For this review, take the finished solid that the model builds, in its own axes (mm). Face numbers are marked on the shaded views. A direction names the side the tool comes from. Coordinates: 2 decimals unless noted, no trailing zeros. Loops run counter-clockwise (first coordinate to the right, second up) from the corner with the lowest first, then second, coordinate; pieces in that order, holes last. Notation, with made-up numbers: (81, -34) -> (85, -34) arc R8 cw to (85, -28) -> close; hole circle Ø7 at (-36.5, 36). An arc over 180 degrees is marked (long way). Answer in a Markdown table with one row per item.
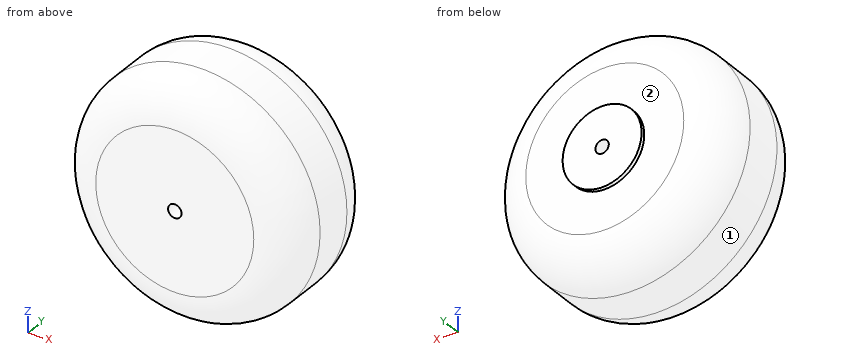
from build123d import *

# Parameters (mm, degrees)
CYLINDER014_R          = 1.7
CYLINDER014_DEPTH      = 31
CYLINDER014_ROLL_ANGLE = 90
CYLINDER012_R          = 30
CYLINDER012_DEPTH      = 30
CYLINDER012_ROLL_ANGLE = 90
CYLINDER013_R          = 10
CYLINDER013_DEPTH      = 31
CYLINDER013_ROLL_ANGLE = 90
FILLET004_R            = 10


with BuildPart() as cilindro014:
    # Cylinder014 → Cylinder014 (new body)
    with BuildSketch(Plane.XY):
        Circle(CYLINDER014_R)
    extrude(amount=CYLINDER014_DEPTH)


with BuildPart() as cilindro014_1:
    # Cylinder014 roll: moved
    add(cilindro014.part.rotate(Axis((0, 0, 0), (1, 0, 0)), CYLINDER014_ROLL_ANGLE))


with BuildPart() as cilindro014_2:
    # Cylinder014 placement: moved
    add(cilindro014_1.part.moved(Location((220, 89, -34.5))))


with BuildPart() as cilindro012:
    # Cylinder012 → Cylinder012 (new body)
    with BuildSketch(Plane.XY):
        Circle(CYLINDER012_R)
    extrude(amount=CYLINDER012_DEPTH)


with BuildPart() as cilindro012_1:
    # Cylinder012 roll: moved
    add(cilindro012.part.rotate(Axis((0, 0, 0), (1, 0, 0)), CYLINDER012_ROLL_ANGLE))


with BuildPart() as cilindro012_2:
    # Cylinder012 placement: moved
    add(cilindro012_1.part.moved(Location((220, 89, -34.5))))


with BuildPart() as fillet004:
    # Cylinder013 → Cylinder013 (new body)
    with BuildSketch(Plane.XY):
        Circle(CYLINDER013_R)
    extrude(amount=CYLINDER013_DEPTH)


with BuildPart() as fillet004_1:
    # Cylinder013 roll: moved
    add(fillet004.part.rotate(Axis((0, 0, 0), (1, 0, 0)), CYLINDER013_ROLL_ANGLE))


with BuildPart() as fillet004_2:
    # Cylinder013 placement: moved
    add(fillet004_1.part.moved(Location((220, 89, -34.5))))

    # Fusion015: union Cilindro012
    add(cilindro012_2.part)

    # Cut008: cut Cilindro014
    add(cilindro014_2.part, mode=Mode.SUBTRACT)

    # Fillet004
    fillet004_edges = [fillet004_2.edges().sort_by_distance(p)[0] for p in [
        (190, 59, -34.5),
        (190, 89, -34.5),
    ]]
    fillet(fillet004_edges, radius=FILLET004_R)


with BuildPart() as part_mirroring001:
    # Part__Mirroring001: instance of Fillet004
    add(fillet004_2.part.mirror(Plane(origin=(220, -4e-06, -34.499992), x_dir=(1, 0, 0), z_dir=(0, 1, 0))))


solid = part_mirroring001.part
Item 1: Take a section at A-A, the plane z = -34.5. State the section outline as (x, y) points.
Worked answers:
| item | result |
|---|---|
| outline | (190, -79) arc R10 ccw to (200, -89) -> (218.3, -89) -> (218.3, -58) -> (210, -58) -> (210, -59) -> (200, -59) arc R10 ccw to (190, -69) -> close; (221.7, -89) -> (240, -89) arc R10 ccw to (250, -79) -> (250, -69) arc R10 ccw to (240, -59) -> (230, -59) -> (230, -58) -> (221.7, -58) -> close |
Item 2: Take a section at C-C, the plane y = -66. State the section outline as (x, z) points, and give its area (3 significant figures).
Worked answers:
| item | result |
|---|---|
| outline | circle Ø59.08 at (220, -34.5); hole circle Ø3.4 at (220, -34.5) |
| area | 2,730 mm² |
Item 3: For L1, parallel to Z at x = 220, y = -68.5; L2, parallel to Z at x = 220, y = -80; L3, parallel to X at y = -82, z = -34, list the stretches that pass through material, from the lowest coordinate up.
Worked answers:
| item | result |
|---|---|
| L1 | -64.49 to -36.2, -32.8 to -4.51 |
| L2 | -64.45 to -36.2, -32.8 to -4.55 |
| L3 | 190.46 to 218.38, 221.62 to 249.54 |
Item 4: For the marked faces 1 and 2, list the 3-axis set-ups (+Z, -Z, +X, -X, +Y, -Y) from which the entire face can be reached by the end or side of a thin tool; tool diameter is ignored.
Worked answers:
| item | result |
|---|---|
| face 1 | +Y, -Y |
| face 2 | +Y |
Item 5: Insertion check: pin 1 (1.5 mm diameter, centred on x = 241, z = -18, fed in from -Y); pin 2 (4 mm diameter, centred on x = 204.5, y = -83, fed in from -Z); pin 3 (2 mm diameter, centred on y = -69, z = -52.5, fed in from +X). Each pin has a flat end and moves straight along its axis. Give the tip position at first contact, or say it passes through.
Worked answers:
| item | result |
|---|---|
| pin 1 | y = -87.03 |
| pin 2 | z = -60.64 |
| pin 3 | x = 244.72 |
Item 6: Take a section at B-B, the plane x = 220. State the section outline as (y, z) points.
Worked answers:
| item | result |
|---|---|
| outline | (-89, -54.5) arc R10 ccw to (-79, -64.5) -> (-69, -64.5) arc R10 ccw to (-59, -54.5) -> (-59, -44.5) -> (-58, -44.5) -> (-58, -36.2) -> (-89, -36.2) -> close; (-89, -32.8) -> (-58, -32.8) -> (-58, -24.5) -> (-59, -24.5) -> (-59, -14.5) arc R10 ccw to (-69, -4.5) -> (-79, -4.5) arc R10 ccw to (-89, -14.5) -> close |
